CAD build for the part. Positions are in the model's coordinates, mm. A direction names the side the tool comes from. Round coordinates to 2 decimals unless told otherwise and drop trailing zeros. Write each loop counter-clockwise with the first axis right and the second up, starting at its lowest first coordinate (ties: lowest second). Pieces come first, ordered by that corner, then holes. Notation, with made-up numbers: (28.25, 72.5) - (65.25, 72.5) arc R17 ccw to (65.25, 103.5) - close; hole circle Ø1 at (50, 51.25). An arc over 180 degrees is marked (long way). Use one line per item in the form item = value. Start each with the question number.
Item 1: Tool access for faces 1 (the flat face through (-20.5, 2, 22)), 2 (the flat face through (-21, 3, 21)), 3 (the flat face through (-1.5, 2, 23)), 4 (the flat face through (-12, 0, 23)), 5 (the flat face through (-12, 2, 1.5)): list every direction of +Z, -Z, +X, -X, +Y, -Y with a clear straight run to the whole face (end or side of a thin tool).
Item 2: Band-saw the part on B-B, the plane z = 10.5. List the corners of the cut face in (x, y).
Item 3: Drill centre lines: L1, parallel to X at y = 2.85, z = 31; L2, parallel to Z at x = -20.25, y = 2.6; L3, parallel to Y at x = -15, z = 7. Where is each one in solid material? Low to high.
Item 4: Pull direction Z, two halves, no side cores. Call faces 6 (the flat face through (-12, 2, 44)), 7 (the flat face through (-3, 2, 23)), 8 (the flat face through (-22, 2, 22)): +Z half, -Z half, draft (parallel to the pull), parting line (faces both ways), or undercut.
Item 5: Pin check, flat tips, straight feed: pin 1 (1.5 mm diameter, centred on y = 2.5, z = 38, fed in from -X); pin 2 (0.8 mm diameter, centred on y = 2.5, z = 26, fed in from +X); pin 3 (1.2 mm diameter, centred on x = -7.5, y = 2.5, fed in from +Z). Stop position of each tip, or through.
Item 6: Band-saw the part on C-C, the plane y = 2.5. List the corners of the cut face in (x, z).
Item 7: Band-saw the part on D-D, the plane x = -2.25. List the corners of the cut face in (y, z), and give its area (3 significant figures).
Item 8: Band-saw the part on A-A, the plane x = -9. List the corners of the cut face in (y, z).
Autodesk Inventor part; units mm, degrees
ref_plane "YZ Plane" through (0, 0, 0) normal (1, 0, 0) x (0, 1, 0)
ref_plane "XZ Plane" through (0, 0, 0) normal (0, 1, 0) x (-1, 0, 0)
ref_plane "XY Plane" through (0, 0, 0) normal (0, 0, 1) x (1, 0, 0)
sketch "Szkic1" plane through (0, 0, 0) normal (0, 1, 0) x (-1, 0, 0)
  line L0 (0, 0) -> (23.5, 0)
  line L1 (23.5, 0) -> (23.5, 45.5)
  line L2 (23.5, 45.5) -> (0, 45.5)
  line L3 (0, 45.5) -> (0, 0)
  dimension "d0" = 23.5
  dimension "d1" = 45.5
extrude "Wyciągnięcie proste1" add sketch "Szkic1" along normal blind 1.5
sketch "Szkic2" plane through (0, 1.5, 0) normal (0, 1, 0) x (1, 0, 0)
  line L0 (-23.5, 0) -> (-23.5, -45.5) construction
  line L1 (-23.5, -45.5) -> (-22, -45.5) construction
  line L2 (-23.5, -45.5) -> (0, -45.5) construction
  line L3 (-22, -45.5) -> (-22, -44) construction
  line L4 (-22, -44) -> (-1.5, -44)
  line L5 (-1.5, -44) -> (-1.5, -1.5)
  line L6 (-1.5, -1.5) -> (-22, -1.5)
  line L7 (-22, -1.5) -> (-22, -44)
  line L8 (-22, -44) -> (-22, -42.5) construction
  line L9 (-22, -42.5) -> (-20.5, -42.5) construction
  line L10 (-1.5, -1.5) -> (-3, -1.5) construction
  line L11 (-3, -1.5) -> (-3, -3) construction
  line L12 (-20.5, -42.5) -> (-3, -42.5)
  line L13 (-3, -42.5) -> (-3, -3)
  line L14 (-3, -3) -> (-20.5, -3)
  line L15 (-20.5, -3) -> (-20.5, -42.5)
  point P0 (0, 0)
  dimension "d4" = 1.5
  dimension "d5" = 1.5
  dimension "d6" = 20.5
  dimension "d7" = 42.5
  dimension "d8" = 1.5
  dimension "d9" = 1.5
  dimension "d10" = 1.5
  dimension "d11" = 1.5
extrude "Wyciągnięcie proste2" add sketch "Szkic2" along normal blind 1.5
properties part number "gora"
Determined:
q1.face_1 = +Y
q1.face_2 = +Z, -Z, +X, -X, +Y
q1.face_3 = +Z, -Z, +X, +Y
q1.face_4 = +Z, -Z, +X, -X, -Y
q1.face_5 = -Z, +X, -X, +Y
q2.outline = (-23.5, 0) - (0, 0) - (0, 1.5) - (-1.5, 1.5) - (-1.5, 3) - (-3, 3) - (-3, 1.5) - (-20.5, 1.5) - (-20.5, 3) - (-22, 3) - (-22, 1.5) - (-23.5, 1.5) - close
q3.L1 = -22 to -20.5, -3 to -1.5
q3.L2 = 1.5 to 3, 42.5 to 44
q3.L3 = 0 to 1.5
q4.face_6 = +Z half
q4.face_7 = undercut
q4.face_8 = draft
q5.pin_1 = -22
q5.pin_2 = -1.5
q5.pin_3 = 44
q6.outline = (-22, 1.5) - (-1.5, 1.5) - (-1.5, 44) - (-22, 44) - close; hole (-20.5, 3) - (-3, 3) - (-3, 42.5) - (-20.5, 42.5) - close
q7.outline = (0, 0) - (1.5, 0) - (1.5, 1.5) - (3, 1.5) - (3, 44) - (1.5, 44) - (1.5, 45.5) - (0, 45.5) - close
q7.area = 132 mm²
q8.outline = (0, 0) - (1.5, 0) - (1.5, 1.5) - (3, 1.5) - (3, 3) - (1.5, 3) - (1.5, 42.5) - (3, 42.5) - (3, 44) - (1.5, 44) - (1.5, 45.5) - (0, 45.5) - close
